CAD build for the part. Positions are in the model's coordinates, mm. Face numbers are marked on the shaded views. A direction names the side the tool comes from. Give positions to 0.01 mm unless a question says otherwise; leave off trailing zeros. Order: outer loops, then holes, each group sorted by start corner. A loop starts at its lowest first (then second) coordinate and runs counter-clockwise, first axis right, second up.
Item 1: Band-saw the part on D-D on x = -2.1. Give the cut face in (y, z), plus the area to 3 significant figures.
Item 2: Which spindle directions (+Z, -Z, +X, -X, +Y, -Y) get a long thin tool onto all of the face, cutting with end or side? Do the marked faces 1 and 2. Say none if no direction does.
Item 3: Wall check: L1, parallel to Z at x = 0, y = -24; L2, parallel to X at y = -8.75, z = -1; L3, parallel to X at y = -9, z = 0.6. Give the ranges that are in metal, low to high.
Item 4: Band-saw the part on C-C on x = 0. Give the cut face in (y, z).
Item 5: Flat gauge pins, fed straight in: P1, Ø0.6, axis at y = -7, z = -0.5, coming from the +X side; P2, Ø0.6, axis at x = -2, y = -17, coming from the +Z side; P3, Ø1.5, axis at x = 2, y = -2.5, coming from the +Z side. Where does each tip first touch, or does it go through?
Item 6: Band-saw the part on B-B on y = -4.25. Give the cut face in (x, z).
Item 7: Band-saw the part on A-A on z = -0.3. Give the cut face in (x, y).
Item 8: Two-plate mould, pull along X, no slides. Class the marked faces 3, 4 and 5: released by +X, released by -X, zero draft, split by the parting line, or undercut.
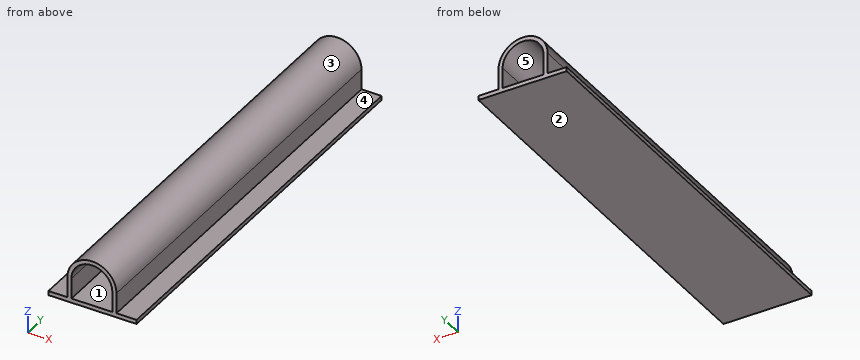
```python
from build123d import *

# Parameters (mm, degrees)
F0_W     = 0.25
F0_H     = 1.25
F1_DEPTH = 25


# Not quite as in the source:
# - a feature names something its author has since deleted; it is built from what else it names


with BuildPart() as f1:
    # F0 (on Front) → F1 (new body)
    with BuildSketch(Plane.XZ):
        with BuildLine():
            ThreePointArc((-1.25, 0), (0, 1.25), (1.25, 0))
            Line((1.25, 0), (1.5, 0))
            ThreePointArc((1.5, 0), (0, 1.5), (-1.5, 0))
            Line((-1.5, 0), (-1.25, 0))
        make_face()
        with Locations((1.375, -0.625)):
            Rectangle(F0_W, F0_H)
        with Locations((-1.375, -0.625)):
            Rectangle(F0_W, F0_H)
        Polygon((1.5, -1.25), (1.25, -1.25), (-1.25, -1.25), (-1.5, -1.25), (-2.6555589866, -1.25), (-2.6555589866, -1.5083510661), (2.7294615284, -1.5083510661), (2.7294615284, -1.25), align=None)
    extrude(amount=F1_DEPTH)


solid = f1.part
```
The answers:
1. outline: (-25, -1.51) - (0, -1.51) - (0, -1.25) - (-25, -1.25) - close
1. area: 6.46 mm2
2. face 1: +Y, -Y
2. face 2: -Z, +X, -X, +Y, -Y
3. L1: z = -1.51 to -1.25, 1.25 to 1.5
3. L2: x = -1.5 to -1.25, 1.25 to 1.5
3. L3: x = -1.37 to -1.1, 1.1 to 1.37
4. outline: (-25, -1.51) - (0, -1.51) - (0, -1.25) - (-25, -1.25) - close; (-25, 1.25) - (0, 1.25) - (0, 1.5) - (-25, 1.5) - close
5. P1: stops at x = 1.5
5. P2: stops at z = -1.25
5. P3: stops at z = 0.83
6. outline: (-2.66, -1.51) - (2.73, -1.51) - (2.73, -1.25) - (1.5, -1.25) - (1.5, 0) arc R1.5 ccw to (-1.5, 0) - (-1.5, -1.25) - (-2.66, -1.25) - close; hole (-1.25, -1.25) - (1.25, -1.25) - (1.25, 0) arc R1.25 ccw to (-1.25, 0) - close
7. outline: (-1.5, -25) - (-1.25, -25) - (-1.25, 0) - (-1.5, 0) - close; (1.25, -25) - (1.5, -25) - (1.5, 0) - (1.25, 0) - close
8. face 3: split by the parting line
8. face 4: zero draft
8. face 5: undercut
